Check sheet for the modelled part. Datum: model origin and axes. Units: mm. Face numbers are marked on the shaded views. A direction names the side the tool comes from. Give positions to 0.01 mm unless a question says otherwise; leave off trailing zeros. Loops run counter-clockwise (first coordinate to the right, second up) from the corner with the lowest first, then second, coordinate; pieces in that order, holes last. Notation, with made-up numbers: (64, 43.25) -> (114, 43.25) arc R8 cw to (114, 57.25) -> close; hole circle Ø6 at (-40, 88). An arc over 180 degrees is marked (long way). Write each question's results on one line, items separated by ' | '. Start each with the question number.
1. Cross-section at A-A on z = 5.5. Record the boundary of the cut face in (x, y) (3 decimals).
2. Material ranges on L1, parallel to Z at x = -27.5, y = 33 (3 decimals); L2, parallel to Y at x = 18, z = 31; L3, parallel to X at y = 35.5, z = 3.5 (3 decimals), recorded low to high. Write a range as from..to.
3. Mould release check, pull along X, two halves, no side actions. Record for the marked faces 1, 2 and 3: +X half, -X half, draft (parallel to the pull), parting line (faces both ways), or undercut.
4. Tool access check on the marked faces 4, 5, 6 and 7. Record the directions out of +Z, -Z, +X, -X, +Y, -Y that give a thin tool (end or side, any length) a straight path to the whole face; none if there is none.
5. Gauge pin test, flat ends, axial feed: pin 1 Ø15.5 at (x, z) = (69, 28) entering from -Y; pin 2 Ø6 at (y, z) = (-17, 45) entering from -X; pin 3 Ø14.5 at (x, y) = (65.5, -5.5) entering from -Z; pin 4 Ø11 at (y, z) = (16.5, 3) entering from +X (3 decimals). Record the tip position at first contact, or that the pin passes through.
6. Cross-section at B-B on y = -35.5. Record the boundary of the cut face in (x, z) (3 decimals).
from build123d import *

# Parameters (mm, degrees)
F1_DEPTH = 63.5
F2_DEPTH = 25.4
F3_DEPTH = 7.9375
F5_R     = 6.35


with BuildPart() as f1:
    # F0 (on Front) → F1 (new body, symmetric)
    with BuildSketch(Plane.XZ):
        Polygon((-41.275, -9.525), (41.275, -9.525), (41.275, 9.525), (22.225, 9.525), (-41.275, 9.525), align=None)
    extrude(amount=F1_DEPTH, both=True)

    # F0 (on Front) → F2 (join, symmetric)
    with BuildSketch(Plane.XZ):
        Polygon((60.325, 61.9252), (60.325, 42.8752), (85.7480703479, 42.8752), (85.8401063105, 61.9252), align=None)
        with BuildLine():
            Line((22.225, 9.525), (41.275, 9.525))
            Line((41.275, 9.525), (41.275, 27.0002))
            ThreePointArc((41.275, 27.0002), (45.9246798487, 38.2255201513), (57.15, 42.8752))
            Line((57.15, 42.8752), (60.325, 42.8752))
            Line((60.325, 42.8752), (60.325, 61.9252))
            Line((60.325, 61.9252), (57.15, 61.9252))
            add(Edge.make_bspline(
                [(56.356848483, 61.9161925488), (56.6214024157, 61.9201926701), (56.8857897727, 61.9231977078), (57.15, 61.9252)],
                knots=[110.870288539, 110.870288539, 110.870288539, 110.870288539, 111.5045361635, 111.5045361635, 111.5045361635, 111.5045361635], degree=3))
            ThreePointArc((56.356848483, 61.9161925488), (32.1754485352, 51.4138724835), (22.225, 27.0002))
            Line((22.225, 27.0002), (22.225, 9.525))
        make_face()
    extrude(amount=F2_DEPTH, both=True)

    # F0 (on Front) → F3 (join, symmetric)
    with BuildSketch(Plane.XZ):
        with BuildLine():
            add(Edge.make_bspline(
                [(-41.275, 9.525), (-41.2244558949, 30.1107989648), (10.1112344326, 61.2169473646), (56.356848483, 61.9161925488)],
                knots=[0, 0, 0, 0, 110.870288539, 110.870288539, 110.870288539, 110.870288539], degree=3))
            Line((-41.275, 9.525), (22.225, 9.525))
            Line((22.225, 9.525), (22.225, 27.0002))
            ThreePointArc((22.225, 27.0002), (32.1754485352, 51.4138724835), (56.356848483, 61.9161925488))
        make_face()
    extrude(amount=F3_DEPTH, both=True)

    # F0 (on Front) → F4 (revolve)
    with BuildSketch(Plane.XZ):
        Polygon((85.8401063105, 61.9252), (85.7480703479, 42.8752), (85.725, 38.1), (111.125, 38.1), (111.125, 66.675), (85.8630539438, 66.675), align=None)
    revolve(axis=Axis((85.7940269719, 0, 52.3875), (0.0048312277, 0, 0.9999883296)))

    # F5
    f5_edges = [f1.edges().sort_by_distance(p)[0] for p in [
        (41.275, -63.5, 0),
        (-41.275, -63.5, 0),
        (41.275, 63.5, 0),
        (-41.275, 63.5, 0),
    ]]
    fillet(f5_edges, radius=F5_R)


solid = f1.part
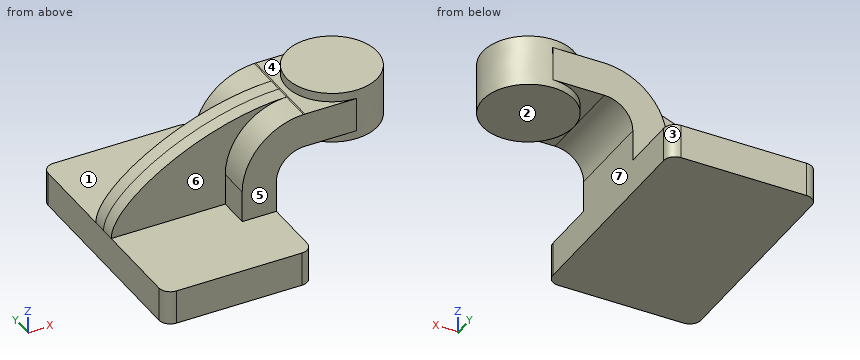
Geometry says:
1) outline: (-41.275, -57.15) arc R6.35 ccw to (-34.925, -63.5) -> (34.925, -63.5) arc R6.35 ccw to (41.275, -57.15) -> (41.275, 57.15) arc R6.35 ccw to (34.925, 63.5) -> (-34.925, 63.5) arc R6.35 ccw to (-41.275, 57.15) -> close
2) L1: -9.525..9.525 | L2: -7.94..7.94 | L3: -41.275..41.275
3) face 1: draft | face 2: undercut | face 3: +X half
4) face 4: +Z, -X | face 5: +Z, +X, -X, -Y | face 6: +Z, -X, -Y | face 7: -Z, +X, +Y, -Y
5) pin 1: through | pin 2: x = 25.61 | pin 3: z = 38.23 | pin 4: x = 41.275
6) outline: (-41.275, -9.525) -> (41.275, -9.525) -> (41.275, 9.525) -> (-41.275, 9.525) -> close
